Autodesk Inventor part; units mm, degrees
ref_plane "YZ Plane" through (0, 0, 0) normal (1, 0, 0) x (0, 1, 0)
ref_plane "XZ Plane" through (0, 0, 0) normal (0, 1, 0) x (-1, 0, 0)
ref_plane "XY Plane" through (0, 0, 0) normal (0, 0, 1) x (1, 0, 0)
sketch "Sketch1" plane through (0, 0, 0) normal (0, 0, 1) x (1, 0, 0)
  circle A0 centre (-6.6643, 9.7203) radius 7.5
  line L0 (-9.6643, 9.7203) -> (-3.6643, 9.7203)
  line L1 (-3.6643, 9.7203) -> (-3.6643, -10.5455)
  line L2 (-3.6643, -10.5455) -> (-9.6643, -10.5455)
  line L3 (-9.6643, -10.5455) -> (-9.6643, 9.7203)
  line L4 (-21.6643, -10.5455) -> (8.3357, -10.5455)
  line L5 (8.3357, -10.5455) -> (8.3357, -14.5455)
  line L6 (8.3357, -14.5455) -> (-21.6643, -14.5455)
  line L7 (-21.6643, -14.5455) -> (-21.6643, -10.5455)
  point P0 (0, 0)
  point P1 (0, 0)
  dimension "d0" = 15
  dimension "d1" = 6
  dimension "d2" = 4
  dimension "d3" = 30
  dimension "d4" = 12
  dimension "d5" = 3
  dimension "d6" = 3
  dimension "d7" = 12
  dimension "d8" = 0
extrude "Extrusion1" add sketch "Sketch1" along normal blind 200
equation "\"d4\" = d7"
properties part number "z rail"
Here's how the part is built. I have some questions about the finished solid (model axes, mm). A direction names the side the tool comes from. Give positions to 0.01 mm unless a question says otherwise; leave off trailing zeros. Loops run counter-clockwise (first coordinate to the right, second up) from the corner with the lowest first, then second, coordinate; pieces in that order, holes last. Notation, with made-up numbers: M 50.25,56.25 L 81.25,56.25 A8 ccw 81.25,64.25 Z; hole C -10.75,62 d6. An arc over 180 degrees is marked long. Use one line per item in the form item = value. Start each with the question number.
Q1. If we section it at B-B (z = 166.5): Write out the boundary of the cut face in (x, y), then the cut area to 3 significant figures.
Q2. Will these pins go through, and if not, where does the flat tip stop? pin 1 Ø3 at (x, z) = (-3, 94.5) entering from +Y; pin 2 Ø10 at (x, y) = (-14, -5.5) entering from +Z; pin 3 Ø6.5 at (y, z) = (-4.5, 105) entering from +X; pin 4 Ø5 at (x, y) = (-16, -7) entering from -Z.
Q3. If we section it at C-C (y = -8.5): Write out the boundary of the cut face in (x, z), then the cut area to 3 significant figures.
Q4. I need wall thicknesses on line 1 along Y through (x, z) = (-16.25, 51.5); line 2 along Y through (x, z) = (-6.5, 151.5); line 3 along X through (y, z) = (-6.5, 148). Which ranges of each line are inside material? Lowest first, please.
Q5. If we section it at D-D (y = 7.5): Write out the boundary of the cut face in (x, z), then the cut area to 3 significant figures.
Q6. Thinking about a two-plate mould opening in Y: for faces 4 (the flat face through (-21.664, -13, 99)), 5 (the cylindrical face through (-6.951, 17.215, 98.6)), 6 (the flat face through (-6, -14.546, 99)), which applies, +Y half, -Y half, draft (parallel to the pull), parting line (faces both ways), or undercut?
Q7. Which directions (+Z, -Z, +X, -X, +Y, -Y) give clear straight access to the entire face, cutting with the end or side of a thin tool? Please do faces 1 (the flat face through (2, -10.546, 99)), 2 (the flat face through (-16, -10.546, 99)), 3 (the flat face through (-7, -1, 200)).
Q8. If we section it at A-A (x = -12.5): Write out the boundary of the cut face in (y, z).
Taken from the geometry:
q1.outline = M -21.66,-14.55 L 8.34,-14.55 L 8.34,-10.55 L -3.66,-10.55 L -3.66,2.85 A7.5 ccw long -9.66,2.85 L -9.66,-10.55 L -21.66,-10.55 Z
q1.area = 375 mm^2
q2.pin_1 = 16.9
q2.pin_2 = 200
q2.pin_3 = -3.66
q2.pin_4 = through
q3.outline = M -9.66,0 L -3.66,0 L -3.66,200 L -9.66,200 Z
q3.area = 1,200 mm^2
q4.line_1 = -14.55 to -10.55
q4.line_2 = -14.55 to 17.22
q4.line_3 = -9.66 to -3.66
q5.outline = M -13.83,0 L 0.5,0 L 0.5,200 L -13.83,200 Z
q5.area = 2,870 mm^2
q6.face_4 = draft
q6.face_5 = undercut
q6.face_6 = -Y half
q7.face_1 = +Z, -Z, +X
q7.face_2 = +Z, -Z, -X
q7.face_3 = +Z, +X, -X, +Y, -Y
q8.outline = M -14.55,0 L -10.55,0 L -10.55,200 L -14.55,200 Z; M 5.01,0 L 14.43,0 L 14.43,200 L 5.01,200 Z
